from build123d import *

# Parameters (mm, degrees)
SKETCH5_R                       = 11.25
SKETCH5_R_2                     = 8.75
BOSS_EXTRUDE3_DEPTH             = 50
SKETCH6_R                       = 8.75
BOSS_EXTRUDE4_DEPTH             = 5
FILLET1_R                       = 0.5
BOSS_EXTRUDE6_REACH             = 62.069
BOSS_EXTRUDE6_END_RADIUS        = 11.25
SKETCH16_R                      = 6.25
CBORE_FOR_M4_SBHCS1_D           = 3
CBORE_FOR_M4_SBHCS1_DEPTH       = 10
CBORE_FOR_M4_SBHCS1_CBORE_D     = 8.6
CBORE_FOR_M4_SBHCS1_CBORE_DEPTH = 2.2
CBORE_FOR_M4_SBHCS1_TIP         = 0.901290929
CUT_EXTRUDE1_DEPTH              = 55.90522149
CUT_EXTRUDE1_DEPTH_BACK         = 55.90522149
SKETCH11_W                      = 2.25
SKETCH11_H                      = 15
M4X0_7_TAPPED_HOLE1_D           = 3.3
M4X0_7_TAPPED_HOLE1_DEPTH       = 10.1
M4X0_7_TAPPED_HOLE1_TIP         = 0.991420021
FILLET3_R                       = 1


with BuildPart() as part:
    # Sketch5 → Boss-Extrude3 (new body)
    with BuildSketch(Plane(origin=(0, 0, 0), x_dir=(1, 0, 0), z_dir=(0, 1, 0))):
        with Locations(Location((0, 0, 0), (0, 0, 270))):
            Circle(SKETCH5_R)
        with Locations(Location((0, 0, 0), (0, 0, 270))):
            Circle(SKETCH5_R_2, mode=Mode.SUBTRACT)
    extrude(amount=BOSS_EXTRUDE3_DEPTH)

    # Sketch6 → Boss-Extrude4 (add)
    with BuildSketch(Plane.XZ):
        Polygon((0, 14.43375673), (-12.5, 7.216878365), (-12.5, -7.216878365), (0, -14.43375673), (12.5, -7.216878365), (12.5, 7.216878365), align=None)
        with Locations(Location((0, 0, 0), (0, 0, 90))):
            Circle(SKETCH6_R, mode=Mode.SUBTRACT)
    extrude(amount=-BOSS_EXTRUDE4_DEPTH)

    # Fillet1
    fillet1_edges = [part.edges().sort_by_distance(p)[0] for p in [
        (0, 5, -11.25),
        (6.25, 0, 10.825317547),
        (-6.25, 0, 10.825317547),
        (-12.5, 0, 0),
        (-6.25, 0, -10.825317547),
        (6.25, 0, -10.825317547),
        (12.5, 0, 0),
        (6.25, 5, 10.825317547),
        (12.5, 5, 0),
        (6.25, 5, -10.825317547),
        (-6.25, 5, -10.825317547),
        (-12.5, 5, 0),
        (-6.25, 5, 10.825317547),
        (0, 50, -11.25),
        (0, 50, -8.75),
    ]]
    fillet(fillet1_edges, radius=FILLET1_R)

    # Boss-Extrude6: up to this cylinder (the profile starts outside it)
    boss_extrude6_end = Plane(origin=(0, 15, 0), z_dir=(0, -1, 0)) * Cylinder(BOSS_EXTRUDE6_END_RADIUS, 147.638, mode=Mode.PRIVATE)
    # Sketch16 → Boss-Extrude6 (add, up to the surface)
    with BuildSketch(Plane(origin=(-17.5, 0, 0), x_dir=(0, 0, -1), z_dir=(1, 0, 0)), mode=Mode.PRIVATE) as boss_extrude6_sk1:
        with Locations(Location((0, 15, 0), (0, 0, 180))):
            Circle(SKETCH16_R)
    boss_extrude6_tool1 = extrude(boss_extrude6_sk1.sketch, amount=BOSS_EXTRUDE6_REACH, mode=Mode.PRIVATE) - boss_extrude6_end
    add(boss_extrude6_tool1.solids().sort_by_distance((-17.5, 15, 0))[0])

    # CBORE for M4 SBHCS1
    with Locations(Plane.ZY.offset(17.5)):
        with Locations((0, 15)):
            CounterBoreHole(CBORE_FOR_M4_SBHCS1_D / 2, CBORE_FOR_M4_SBHCS1_CBORE_D / 2, CBORE_FOR_M4_SBHCS1_CBORE_DEPTH, depth=CBORE_FOR_M4_SBHCS1_DEPTH)
            with Locations((0, 0, -(CBORE_FOR_M4_SBHCS1_DEPTH + CBORE_FOR_M4_SBHCS1_TIP / 2))):  # 118° drill point
                Cone(0, CBORE_FOR_M4_SBHCS1_D / 2, CBORE_FOR_M4_SBHCS1_TIP, mode=Mode.SUBTRACT)

    # Sketch11 → Cut-Extrude1 (cut, two sides: drawn at the far end of the back side and taken through both)
    with BuildSketch(Plane(origin=(0, 0, 0), x_dir=(0, 0, -1), z_dir=(1, 0, 0)).offset(-CUT_EXTRUDE1_DEPTH_BACK)):
        with Locations((-10.125, 27.5)):
            Rectangle(SKETCH11_W, SKETCH11_H)
        with Locations((10.125, 27.5)):
            Rectangle(SKETCH11_W, SKETCH11_H)
    extrude(amount=CUT_EXTRUDE1_DEPTH + CUT_EXTRUDE1_DEPTH_BACK, mode=Mode.SUBTRACT)

    # M4x0.7 Tapped Hole1
    with Locations(Plane.ZY.offset(15.3)):
        with Locations((0, 15)):
            Hole(M4X0_7_TAPPED_HOLE1_D / 2, depth=M4X0_7_TAPPED_HOLE1_DEPTH)
            with Locations((0, 0, -(M4X0_7_TAPPED_HOLE1_DEPTH + M4X0_7_TAPPED_HOLE1_TIP / 2))):  # 118° drill point
                Cone(0, M4X0_7_TAPPED_HOLE1_D / 2, M4X0_7_TAPPED_HOLE1_TIP, mode=Mode.SUBTRACT)

    # Fillet3
    fillet3_edges = [part.edges().sort_by_distance(p)[0] for p in [
        (-9.354143467, 15, -6.25),
        (-17.5, 15, -6.25),
    ]]
    fillet(fillet3_edges, radius=FILLET3_R)


solid = part.part
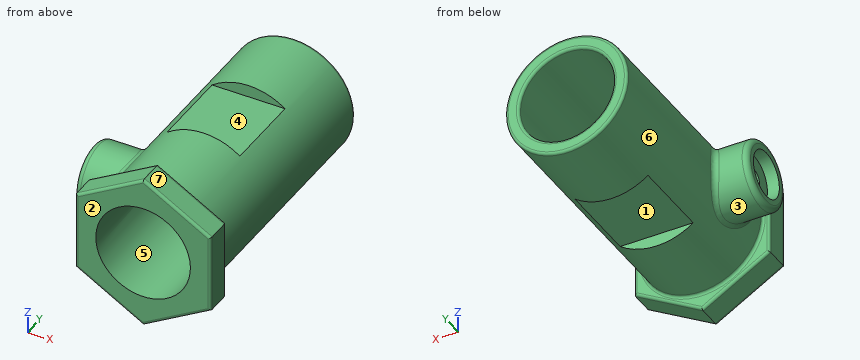
Geometry check sheet. Reference: the model listing, model coordinates, mm. Face numbers are marked on the shaded views. A direction names the side the tool comes from. Give positions to 0.01 mm unless a question says otherwise; leave off trailing zeros. Loops run counter-clockwise (first coordinate to the right, second up) from the corner with the lowest first, then second, coordinate; pieces in that order, holes last. Notation, with made-up numbers: M 74,6 L 123,6 A30 cw 123,44 Z; hole C 82.25,-36.5 d6. An arc over 180 degrees is marked long. Answer as a JSON object with one key per item and string values. Group by question number.
Item 1: Mould release check, pull along Z, two halves, no side actions. Record for the marked faces 5, 6 and 7: pulls with the +Z half, pulls with the -Z half, needs draft (parallel to the pull), parting line crosses it, or undercut.
Item 2: Sectioned sample at B-B on z = 0. Give the number of separate pieces and of enclosed holes in the cut face, plus the area to 3 significant figures.
Item 3: Material ranges on L1, parallel to Y at x = -16.3, z = 0; L2, parallel to X at y = 30, z = 0; L3, parallel to Z at x = -13.75, y = 15, recorded low to high.
Item 4: Gauge pin test, flat ends, axial feed: pin 1 (4.5 mm diameter, centred on y = 3, z = 0.5, fed in from -X); pin 2 (4 mm diameter, centred on x = 1.5, y = 25.5, fed in from +Z); pin 3 (3 mm diameter, centred on y = 11.5, z = -8, fed in from -X). Record the tip position at first contact, or that the pin passes through.
Item 5: Access from +Z, -Z, +X, -X, +Y, -Y to the whole of each face (thin tool, end or side, straight path). Record for the marked faces 1, 2, 3 and 4.
Item 6: Sectioned sample at A-A on y = 33.5. Record the boundary of the cut face in (x, z), plus the area to 3 significant figures.
Findings below:
{
 "1": {"face 5": "undercut", "face 6": "parting line crosses it", "face 7": "pulls with the +Z half"},
 "2": {"separate pieces": "3", "enclosed holes": "0", "area": "300 mm2"},
 "3": {"L1": "8.75 to 10.7, 19.3 to 21.25", "L2": "-11.25 to -8.75, 8.75 to 11.25", "L3": "-6.25 to -1.65, 1.65 to 6.25"},
 "4": {"pin 1": "x = -12.5", "pin 2": "z = 9", "pin 3": "x = -9.18"},
 "5": {"face 1": "-Z, +X, -X", "face 2": "+Z, -Z, +X, -X, -Y", "face 3": "-X", "face 4": "+Z, +X, -X"},
 "6": {"outline": "M -6.75,-9 L 6.75,-9 A11.25 ccw 6.75,9 L -6.75,9 A11.25 ccw Z; hole C 0,0 d17.5", "area": "116 mm2"}
}
